Verification items for this drawing (mm, ordinates from the low corner). A direction names the side the tool comes from. Round coordinates to 2 decimals unless told otherwise and drop trailing zeros. Write each loop counter-clockwise with the first axis right and the second up, starting at its lowest first coordinate (ties: lowest second). Pieces come first, ordered by that corner, then holes. Notation, with made-up numbers: (23, 83.5) -> (30, 83.5) arc R29 ccw to (30, 122.5) -> close; hole circle Ø10 at (40, 7). An arc over 180 degrees is marked (long way). One line per item, written item: value.
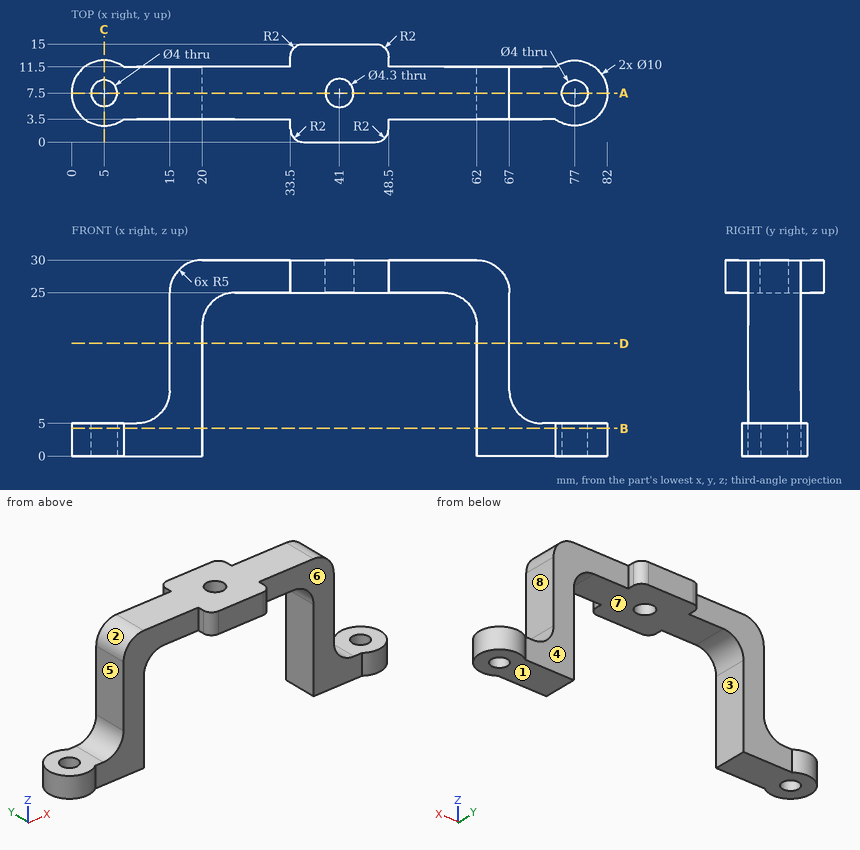
Item 1: Material ranges on line 1 along X through (y, z) = (10.25, 10); line 2 along Y through (x, z) = (5, 1.8); line 3 along X through (y, z) = (6.25, 1), recorded low to high.
Result set:
line 1: 15 to 20, 62 to 67
line 2: 2.5 to 5.5, 9.5 to 12.5
line 3: 0.16 to 3.44, 6.56 to 20, 62 to 75.44, 78.56 to 81.84
Item 2: Release check for a two-part mould opening along X. For the marked faces 1, 2 and 3 record: pulls with the +X half, pulls with the -X half, needs draft (parallel to the pull), parting line crosses it, or undercut.
Result set:
face 1: needs draft
face 2: pulls with the -X half
face 3: undercut
Item 3: Sectioned sample at A-A (y = 7.5). State how many separate pieces and enclosed holes the cut face has, then the cut area to 3 significant figures.
Result set:
separate pieces: 4
enclosed holes: 0
area: 609 mm^2
Item 4: Tool access check on the marked faces 4, 5, 6, 7 and 8. Record the directions out of +Z, -Z, +X, -X, +Y, -Y that give a thin tool (end or side, any length) a straight path to the whole face; none if there is none.
Result set:
face 4: +Z, -Z, +Y
face 5: +Z, -X, +Y, -Y
face 6: +Z, -Z, -Y
face 7: -Z, +Y, -Y
face 8: +Z, +X, +Y, -Y
Item 5: Sectioned sample at B-B (z = 4.25). Enter the section's corners in (x, y), then the cut area to 3 significant figures.
Result set:
outline: (8, 3.5) -> (20, 3.5) -> (20, 11.5) -> (8, 11.5) arc R5 ccw (long way) to start; (62, 3.5) -> (74, 3.5) arc R5 ccw (long way) to (74, 11.5) -> (62, 11.5) -> close; hole circle Ø4 at (5, 7.5); hole circle Ø4 at (77, 7.5)
area: 302 mm^2
Item 6: Sectioned sample at C-C (x = 5). Enter the section's corners in (y, z), then the cut area to 3 significant figures.
Result set:
outline: (2.5, 0) -> (5.5, 0) -> (5.5, 5) -> (2.5, 5) -> close; (9.5, 0) -> (12.5, 0) -> (12.5, 5) -> (9.5, 5) -> close
area: 30.0 mm^2
Item 7: Depth check by flat-ended pin: pin 1 (7.5 mm diameter, centred on x = 22, z = 19.5, fed in from -Y); pin 2 (2.5 mm diameter, centred on y = 9, z = 6, fed in from +X); pin 3 (4 mm diameter, centred on y = 5.5, z = 18.5, fed in from -X). Enter the tip coordinate at first touch or a pass-through.
Result set:
pin 1: y = 3.5
pin 2: x = 81.94
pin 3: x = 15
Item 8: Sectioned sample at D-D (z = 17.25). Enter the section's corners in (x, y), then the cut area to 3 significant figures.
Result set:
outline: (15, 3.5) -> (20, 3.5) -> (20, 11.5) -> (15, 11.5) -> close; (62, 3.5) -> (67, 3.5) -> (67, 11.5) -> (62, 11.5) -> close
area: 80.0 mm^2
